Geometry: final body of the model. Coordinates: model frame, mm. A direction names the side the tool comes from. Give positions to 0.01 mm unless a question says otherwise; leave off trailing zeros. Write each loop counter-clockwise with the first axis right and the second up, starting at its lowest first coordinate (ties: lowest second). Pieces come first, ordered by that corner, then holes. Notation, with made-up numbers: (-34, -1) -> (-23, -1) arc R26 cw to (-23, 28) -> close; hole circle Ø5 at (70, 44.5). An arc over 180 degrees is marked (long way). Answer as a JSON object with one key per item and string values. Group by question number.
(1) Set-up query: faces 1 (the face through (-48, 59, -46.241)), 2 (the face through (-19.513, 59, -3)), 3 (the face through (-48, 9, 38.255)), 4 (the face through (-72, 50, 33.465)). Return all of +Z, -Z, +X, -X, +Y, -Y with unobstructed straight access to the full face (end or side cutting, diameter ignored); none if empty.
(2) Section query B-B on y = 47. Output: boundary loops of the cut face in (x, z), plus the area to 3 significant figures.
(3) Draft query along Y for faces 5 (the face through (-48, 42, -46.241)), 6 (the face through (-48, 0, -5)), 7 (the face through (-48, 43, -5)). Return one class per face: +Y half, -Y half, draft (parallel to the pull), parting line (faces both ways), or undercut.
(4) Material intervals for probe 1 along Y at (x, z) = (-57, 4.5); probe 2 along Z at (x, y) = (-70, 19); probe 3 along Z at (x, y) = (-22.5, 50.5), sorted ascending.
(5) Section query C-C on z = -23. Output: boundary loops of the cut face in (x, y).
(6) Section query D-D on y = 13. Output: boundary loops of the cut face in (x, z).
(7) Contact query for flat-ended pins moving along their axis: pin 1 Ø3 at (y, z) = (43, -28) entering from +X; pin 2 Ø1 at (y, z) = (12.5, -14.5) entering from +X; pin 3 Ø2 at (x, y) = (-71.5, 54) entering from +Z; pin 4 Ø0.6 at (y, z) = (42, -1.5) entering from -X. Output: stop coordinate, or through.
(8) Section query A-A on x = -52. Output: boundary loops of the cut face in (y, z).
from build123d import *

# Parameters (mm, degrees)
SKETCH1_W           = 65
SKETCH1_H           = 95
BOSS_EXTRUDE1_DEPTH = 8
SKETCH2_W           = 55.842972677
SKETCH2_H           = 84.495387978
BOSS_EXTRUDE2_DEPTH = 3
BOSS_EXTRUDE3_DEPTH = 30
SKETCH4_W           = 55.842972677
SKETCH4_H           = 84.495387978
BOSS_EXTRUDE4_DEPTH = 2
BOSS_EXTRUDE5_DEPTH = 15
SKETCH6_W           = 55.842972677
SKETCH6_H           = 84.495387978
BOSS_EXTRUDE6_DEPTH = 2


with BuildPart() as part:
    # Sketch1 → Boss-Extrude1 (new body)
    with BuildSketch(Plane(origin=(0, 0, 0), x_dir=(1, 0, 0), z_dir=(0, 1, 0))):
        with Locations((-47.520746888, 4.139004149)):
            Rectangle(SKETCH1_W, SKETCH1_H)
    extrude(amount=BOSS_EXTRUDE1_DEPTH)

    # Sketch2 → Boss-Extrude2 (add)
    with BuildSketch(Plane(origin=(0, 8, 0), x_dir=(1, 0, 0), z_dir=(0, 1, 0))):
        with Locations((-47.434076541, 3.992818357)):
            Rectangle(SKETCH2_W, SKETCH2_H)
    extrude(amount=BOSS_EXTRUDE2_DEPTH)

    # Sketch3 → Boss-Extrude3 (add)
    with BuildSketch(Plane(origin=(0, 11, 0), x_dir=(1, 0, 0), z_dir=(0, 1, 0))):
        Polygon((-68.533559236, 41.562566991), (-69.361945393, 42.997373903), (-71.018717706, 42.997373903), (-71.847103863, 41.562566991), (-71.018717706, 40.127760079), (-69.361945393, 40.127760079), align=None)
        Polygon((-23.021049218, 41.562566991), (-23.800706777, 42.912973496), (-25.360021896, 42.912973496), (-26.139679455, 41.562566991), (-25.360021896, 40.212160486), (-23.800706777, 40.212160486), align=None)
        Polygon((-22.338848854, -35.42861698), (-23.069777816, -34.162610881), (-24.531635739, -34.162610881), (-25.262564701, -35.42861698), (-24.531635739, -36.694623078), (-23.069777816, -36.694623078), align=None)
        Polygon((-68.533559236, -35.42861698), (-69.361945393, -33.993810068), (-71.018717706, -33.993810068), (-71.847103863, -35.42861698), (-71.018717706, -36.863423892), (-69.361945393, -36.863423892), align=None)
    extrude(amount=BOSS_EXTRUDE3_DEPTH)

    # Sketch4 → Boss-Extrude4 (add)
    with BuildSketch(Plane(origin=(0, 41, 0), x_dir=(1, 0, 0), z_dir=(0, 1, 0))):
        with Locations((-47.434076541, 3.992818357)):
            Rectangle(SKETCH4_W, SKETCH4_H)
    extrude(amount=BOSS_EXTRUDE4_DEPTH)

    # Sketch5 → Boss-Extrude5 (add)
    with BuildSketch(Plane(origin=(0, 43, 0), x_dir=(1, 0, 0), z_dir=(0, 1, 0))):
        Polygon((-69.60558838, 42.92696772), (-70.580160329, 44.614975851), (-72.529304227, 44.614975851), (-73.503876176, 42.92696772), (-72.529304227, 41.238959588), (-70.580160329, 41.238959588), align=None)
        Polygon((-21.4617341, 42.92696772), (-22.290120256, 44.361774631), (-23.94689257, 44.361774631), (-24.775278726, 42.92696772), (-23.94689257, 41.492160808), (-22.290120256, 41.492160808), align=None)
        Polygon((-22.290120256, -33.666923337), (-23.976783563, -33.68418091), (-24.80516972, -35.153502968), (-23.94689257, -36.605567453), (-22.260229263, -36.58830988), (-21.431843106, -35.118987822), align=None)
        Polygon((-69.60558838, -35.153502968), (-70.580160329, -33.465494837), (-72.529304227, -33.465494837), (-73.503876176, -35.153502968), (-72.529304227, -36.8415111), (-70.580160329, -36.8415111), align=None)
    extrude(amount=BOSS_EXTRUDE5_DEPTH)

    # Sketch6 → Boss-Extrude6 (add)
    with BuildSketch(Plane(origin=(0, 58, 0), x_dir=(1, 0, 0), z_dir=(0, 1, 0))):
        with Locations((-47.434076541, 3.992818357)):
            Rectangle(SKETCH6_W, SKETCH6_H)
    extrude(amount=BOSS_EXTRUDE6_DEPTH)


solid = part.part
Answer list:
{
 "1": {"face 1": "-Z, +X, -X, +Y", "face 2": "+Z, -Z, +X, +Y", "face 3": "+Z, +X, -X, +Y", "face 4": "+X, -X"},
 "2": {"outline": "(-73.5, -42.93) -> (-72.53, -44.61) -> (-70.58, -44.61) -> (-69.61, -42.93) -> (-70.58, -41.24) -> (-72.53, -41.24) -> close; (-73.5, 35.15) -> (-72.53, 33.47) -> (-70.58, 33.47) -> (-69.61, 35.15) -> (-70.58, 36.84) -> (-72.53, 36.84) -> close; (-24.81, 35.15) -> (-23.98, 33.68) -> (-22.29, 33.67) -> (-21.43, 35.12) -> (-22.26, 36.59) -> (-23.95, 36.61) -> close; (-24.78, -42.93) -> (-23.95, -44.36) -> (-22.29, -44.36) -> (-21.46, -42.93) -> (-22.29, -41.49) -> (-23.95, -41.49) -> close", "area": "34.3 mm2"},
 "3": {"face 5": "draft", "face 6": "-Y half", "face 7": "undercut"},
 "4": {"probe 1": "0 to 11, 41 to 43, 58 to 60", "probe 2": "-43 to -40.13, 33.99 to 36.86", "probe 3": "-44.36 to -41.49, 33.67 to 36.59"},
 "5": {"outline": "(-80.02, 0) -> (-15.02, 0) -> (-15.02, 8) -> (-19.51, 8) -> (-19.51, 11) -> (-75.36, 11) -> (-75.36, 8) -> (-80.02, 8) -> close; (-75.36, 41) -> (-19.51, 41) -> (-19.51, 43) -> (-75.36, 43) -> close; (-75.36, 58) -> (-19.51, 58) -> (-19.51, 60) -> (-75.36, 60) -> close"},
 "6": {"outline": "(-71.85, -41.56) -> (-71.02, -43) -> (-69.36, -43) -> (-68.53, -41.56) -> (-69.36, -40.13) -> (-71.02, -40.13) -> close; (-71.85, 35.43) -> (-71.02, 33.99) -> (-69.36, 33.99) -> (-68.53, 35.43) -> (-69.36, 36.86) -> (-71.02, 36.86) -> close; (-26.14, -41.56) -> (-25.36, -42.91) -> (-23.8, -42.91) -> (-23.02, -41.56) -> (-23.8, -40.21) -> (-25.36, -40.21) -> close; (-25.26, 35.43) -> (-24.53, 34.16) -> (-23.07, 34.16) -> (-22.34, 35.43) -> (-23.07, 36.69) -> (-24.53, 36.69) -> close"},
 "7": {"pin 1": "x = -19.51", "pin 2": "through", "pin 3": "z = 36.84", "pin 4": "x = -75.36"},
 "8": {"outline": "(0, -51.64) -> (8, -51.64) -> (8, -46.24) -> (11, -46.24) -> (11, 38.25) -> (8, 38.25) -> (8, 43.36) -> (0, 43.36) -> close; (41, -46.24) -> (43, -46.24) -> (43, 38.25) -> (41, 38.25) -> close; (58, -46.24) -> (60, -46.24) -> (60, 38.25) -> (58, 38.25) -> close"}
}
